Autodesk Inventor part; units mm, degrees
ref_plane "YZ Plane" through (0, 0, 0) normal (1, 0, 0) x (0, 1, 0)
ref_plane "XZ Plane" through (0, 0, 0) normal (0, 1, 0) x (-1, 0, 0)
ref_plane "XY Plane" through (0, 0, 0) normal (0, 0, 1) x (1, 0, 0)
sketch "Sketch1" plane through (0, 0, 0) normal (0, 0, 1) x (1, 0, 0)
  line L0 (-47, 6.4) -> (47, 6.4)
  line L1 (47, 6.4) -> (47, -6.4)
  line L2 (47, -6.4) -> (-47, -6.4)
  line L3 (-47, -6.4) -> (-47, 6.4)
  point P0 (0, 0)
  point P1 (-47, 0)
  point P2 (0, 6.4)
  dimension "d0" = 94
  dimension "d1" = 12.8
extrude "Extrusion1" add sketch "Sketch1" along normal blind 16
chamfer "Chamfer1" distance 0.2 angle 45 12 edges at (0, 6.4, 16) (-47, 0, 16) (-47, 6.4, 8) (0, 6.4, 0) (0, -6.4, 16) (0, -6.4, 0) (47, -6.4, 8) (47, 6.4, 8) (47, 0, 16) (47, 0, 0) (-47, 0, 0) (-47, -6.4, 8)
sketch "Sketch2" plane through (-46.8, 6.4, 0.2) normal (0, 1, 0) x (1, 0, 0)
  circle A0 centre (5.3, -2.8) radius 1.5
  circle A1 centre (5.3, -12.8) radius 1.5
  line L0 (0, -15.8) -> (93.6, -15.8)
  line L1 (93.6, 0.2) -> (0, 0.2)
  line L2 (-0.2, 0) -> (-0.2, -15.6)
  line L3 (7.8, 0.2) -> (7.8, -15.8)
  point P0 (46.8, 0.2)
  dimension "d7" = 3
  dimension "d8" = 10
  dimension "d9" = 16
  dimension "d10" = 3
  dimension "d11" = 5.5
  dimension "d12" = 8
extrude "Extrusion2" cut sketch "Sketch2" against normal blind 5
thread "Thread1"
thread "Thread2"
chamfer "Chamfer2" distance 0.2 angle 45 2 edges at (-43, 6.4, 13) (-43, 6.4, 3)
sketch "Sketch3" plane through (-46.8, -6.4, 15.8) normal (0, -1, 0) x (1, 0, 0)
  circle A0 centre (4.8, -7.8) radius 1.6
  circle A1 centre (88.8, -7.8) radius 1.6
  line L0 (0, -15.6) -> (0, 0)
  line L1 (93.6, 0) -> (93.6, -15.6)
  line L2 (-0.2, 0) -> (-0.2, -15.6)
  line L3 (93.8, -15.6) -> (93.8, 0)
  point P0 (46.8, -15.8)
  point P1 (0, -7.8)
  point P2 (93.6, -7.8)
  dimension "d22" = 3.2
  dimension "d23" = 5
  dimension "d24" = 5
extrude "Extrusion3" cut sketch "Sketch3" against normal blind 5
thread "Thread3"
thread "Thread4"
equation "\"d10\" = -0.5 * d8 + 0.5 * d9"
properties part number "Aluminum Mounting Bridge"
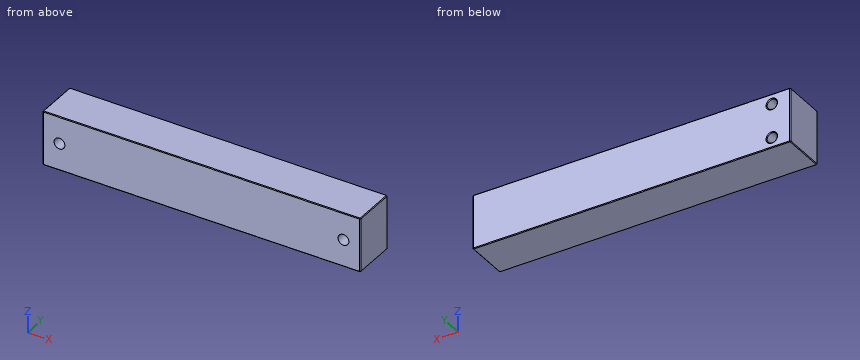
Model file for the job. Use its own axes, mm. Give positions to 0.01 mm unless a question says otherwise; leave off trailing zeros. Order: outer loops, then holes, each group sorted by start corner. A loop starts at its lowest first (then second) coordinate and runs counter-clockwise, first axis right, second up. Notation, with made-up numbers: (84, -21) - (114, -21) arc R13 cw to (114, -3) - close; hole circle Ø5 at (65.5, 45). An arc over 180 degrees is marked (long way). Return JSON: item names as keys, results as strings.
1) Probe line 1 (Z direction, x = -41.5, y = 5.25); line 2 (X direction, y = 2.45, z = 13); line 3 (Z direction, x = -42, y = -4.3). List the from-to ranges inside material, lowest first. Write a range as from..to.
Geometry says:
{"line 1": "0..1.5, 4.5..11.5, 14.5..16", "line 2": "-47..-43, -40..47", "line 3": "0..6.4, 9.6..16"}
2) Cut at A-A, the plane x = 42. Give the cut face in (y, z), plus the area to 3 significant figures.
Geometry says:
{"outline": "(-6.4, 0.2) - (-6.2, 0) - (6.2, 0) - (6.4, 0.2) - (6.4, 15.8) - (6.2, 16) - (-6.2, 16) - (-6.4, 15.8) - (-6.4, 9.6) - (-1.4, 9.6) - (-1.4, 6.4) - (-6.4, 6.4) - close", "area": "189 mm²"}
3) Flat gauge pin, fed straight in: P1, Ø0.9, axis at x = -41, z = 3, coming from the +Y side. Where does the tip first touch, or does it go through?
Geometry says:
{"P1": "y = 1.4"}
4) Cut at B-B, the plane z = 8. Give the cut face in (x, y), plus the area to 3 significant figures.
Geometry says:
{"outline": "(-47, -6.2) - (-46.8, -6.4) - (-43.6, -6.4) - (-43.6, -1.4) - (-40.4, -1.4) - (-40.4, -6.4) - (40.4, -6.4) - (40.4, -1.4) - (43.6, -1.4) - (43.6, -6.4) - (46.8, -6.4) - (47, -6.2) - (47, 6.2) - (46.8, 6.4) - (-46.8, 6.4) - (-47, 6.2) - close", "area": "1,170 mm²"}
